Can you work these out from the model? Positions are in its coordinate system, mm. A direction names the side the tool comes from. Round coordinates to 2 decimals unless told otherwise and drop trailing zeros. Write each loop counter-clockwise with the first axis right and the second up, starting at its lowest first coordinate (ties: lowest second). Pieces come first, ordered by that corner, then holes. Notation, with made-up numbers: (-27.5, 38) -> (18.5, 38) arc R24 cw to (18.5, 57) -> close; hole circle Ø5 at (7.5, -12.5). An arc over 180 degrees is marked (long way). Write item = value, one per line. Start each with the question number.
1) If I drill on line 1 (X direction, y = 1.45, z = -8.25); line 2 (Y direction, x = 12, z = -9.25); line 3 (Y direction, x = 13, z = -3.75), over which ranges is the centre line in solid material (lowest first)?
2) Thinking about a two-plate mould opening in X: for faces 3 (the face through (0, 2, 0.958)), 4 (the face through (13, 1, -8)), 5 (the face through (15.333, 2.007, -11.314)), which applies, +X half, -X half, draft (parallel to the pull), parting line (faces both ways), or undercut?
3) Imagine slicing it at C-C, the plane z = -9.5. Please give me the cut outline in (x, y).
4) Imagine slicing it at B-B, the plane x = 4.5. Please give me the cut outline in (y, z).
5) Imagine slicing it at A-A, the plane y = 0.55. Please give me the cut outline in (x, z).
6) I'm going to push a flat-ended pin straight in: pin 1 (1 mm diameter, centred on y = 1.5, z = -2, fed in from +X). Where does the tip first touch, or does it pass through?
7) For faces 1 (the face through (14.23, 1.76, -8.78)), 2 (the face through (-20.79, 0.45, -9.64)), which set-ups out of +Z, -Z, +X, -X, +Y, -Y let a thin tool reach every point of the face, with its end or its side?
from build123d import *

# Parameters (mm, degrees)
BOSS_EXTRUDE1_DEPTH = 2.5
SKETCH4_R           = 1.78
CUT_EXTRUDE1_DEPTH  = 1.5
FILLET1_R           = 1.5


with BuildPart() as part:
    # Sketch2 → Boss-Extrude1 (new body)
    with BuildSketch(Plane(origin=(0, 0, 0), x_dir=(1, 0, 0), z_dir=(0, 1, 0))):
        Polygon((-21.216153836, 11.741903429), (-21.216153836, 8.241903429), (-7.216153836, -0.958096571), (7.783846164, -0.958096571), (15.783846164, 3.741903429), (15.783846164, 11.741903429), align=None)
    extrude(amount=BOSS_EXTRUDE1_DEPTH)

    # Sketch4 → Cut-Extrude1 (cut)
    with BuildSketch(Plane(origin=(0, 2.5, 0), x_dir=(1, 0, 0), z_dir=(0, 1, 0))):
        with Locations((-17.966153836, 8.241903429)):
            Circle(SKETCH4_R)
        with Locations((12.533846164, 8.241903429)):
            Circle(SKETCH4_R)
    extrude(amount=-CUT_EXTRUDE1_DEPTH, mode=Mode.SUBTRACT)

    # Fillet1
    fillet1_edges = [part.edges().sort_by_distance(p)[0] for p in [
        (15.783846164, 1.25, -11.741903429),
        (15.783846164, 1.25, -3.741903429),
        (7.783846164, 1.25, 0.958096571),
        (-7.216153836, 1.25, 0.958096571),
        (-21.216153836, 1.25, -8.241903429),
        (-21.216153836, 1.25, -11.741903429),
        (15.783846164, 0, -7.741903429),
        (11.783846164, 0, -1.391903429),
        (0.283846164, 0, 0.958096571),
        (-14.216153836, 0, -3.641903429),
        (-21.216153836, 0, -9.991903429),
        (-2.716153836, 0, -11.741903429),
    ]]
    fillet(fillet1_edges, radius=FILLET1_R)


solid = part.part
Reported:
q1.line_1 = -20.98 to -19.75, -16.19 to 10.75, 14.31 to 15.78
q1.line_2 = 0 to 1
q1.line_3 = 0 to 2.5
q2.face_3 = draft
q2.face_4 = undercut
q2.face_5 = +X half
q3.outline = (-21.22, 1.5) arc R1.5 ccw to (-19.72, 0) -> (14.28, 0) arc R1.5 ccw to (15.78, 1.5) -> (15.78, 2.5) -> (13.79, 2.5) -> (13.79, 1) -> (11.27, 1) -> (11.27, 2.5) -> (-16.71, 2.5) -> (-16.71, 1) -> (-19.23, 1) -> (-19.23, 2.5) -> (-21.22, 2.5) -> close
q4.outline = (0, -10.24) arc R1.5 ccw to (1.5, -11.74) -> (2.5, -11.74) -> (2.5, 0.96) -> (1.5, 0.96) arc R1.5 ccw to (0, -0.54) -> close
q5.outline = (-20.88, -10.24) arc R1.16 ccw to (-19.72, -11.4) -> (14.28, -11.4) arc R1.16 ccw to (15.44, -10.24) -> (15.44, -4.6) arc R1.16 ccw to (14.87, -3.6) -> (7.96, 0.46) arc R1.16 ccw to (7.38, 0.62) -> (-6.77, 0.62) arc R1.16 ccw to (-7.4, 0.43) -> (-20.35, -8.08) arc R1.16 ccw to (-20.88, -9.05) -> close
q6.pin_1 = 13.67
q7.face_1 = +Y
q7.face_2 = +Z, -Z, -X, -Y
